Could you check a few things on this model? Use its own coordinates, in mm. Round coordinates to 2 decimals unless told otherwise and drop trailing zeros. Write each loop counter-clockwise with the first axis right and the second up, starting at its lowest first coordinate (ties: lowest second). Pieces come first, ordered by that corner, then holes. Notation, with made-up numbers: (-4, -6.75) -> (39, -6.75) arc R28 ccw to (39, 24.25) -> close; hole circle Ø10 at (-13, -19). An arc over 180 degrees is marked (long way). Return JSON: item names as keys, results as strings.
from build123d import *

# Parameters (mm, degrees)
F0_R     = 1042.9875
F0_R_2   = 6.35
F1_DEPTH = 6.35


with BuildPart() as f1:
    # F0 (on Top) → F1 (new body)
    with BuildSketch(Plane.XY):
        Circle(F0_R)
        with Locations((-534.1764076374, -871.6966720274)):
            Circle(F0_R_2, mode=Mode.SUBTRACT)
        with Locations((-871.6966720274, -534.1764076374)):
            Circle(F0_R_2, mode=Mode.SUBTRACT)
        with Locations((-663.9632122104, -777.4010389312)):
            Circle(F0_R_2, mode=Mode.SUBTRACT)
        with Locations((-777.4010389312, -663.9632122104)):
            Circle(F0_R_2, mode=Mode.SUBTRACT)
        with Locations((-391.2364070784, -944.5282400629)):
            Circle(F0_R_2, mode=Mode.SUBTRACT)
        with Locations((-238.6628677381, -994.1023881186)):
            Circle(F0_R_2, mode=Mode.SUBTRACT)
        with Locations((-80.2126565174, -1019.1984361421)):
            Circle(F0_R_2, mode=Mode.SUBTRACT)
        with Locations((-944.5282400629, -391.2364070784)):
            Circle(F0_R_2, mode=Mode.SUBTRACT)
        with Locations((-994.1023881186, -238.6628677381)):
            Circle(F0_R_2, mode=Mode.SUBTRACT)
        with Locations((-1019.1984361421, -80.2126565174)):
            Circle(F0_R_2, mode=Mode.SUBTRACT)
        with Locations((80.2126565174, -1019.1984361421)):
            Circle(F0_R_2, mode=Mode.SUBTRACT)
        with Locations((238.6628677381, -994.1023881186)):
            Circle(F0_R_2, mode=Mode.SUBTRACT)
        with Locations((391.2364070784, -944.5282400629)):
            Circle(F0_R_2, mode=Mode.SUBTRACT)
        with Locations((534.1764076374, -871.6966720274)):
            Circle(F0_R_2, mode=Mode.SUBTRACT)
        with Locations((663.9632122104, -777.4010389312)):
            Circle(F0_R_2, mode=Mode.SUBTRACT)
        with Locations((777.4010389312, -663.9632122104)):
            Circle(F0_R_2, mode=Mode.SUBTRACT)
        with Locations((871.6966720274, -534.1764076374)):
            Circle(F0_R_2, mode=Mode.SUBTRACT)
        with Locations((944.5282400629, -391.2364070784)):
            Circle(F0_R_2, mode=Mode.SUBTRACT)
        with Locations((994.1023881186, -238.6628677381)):
            Circle(F0_R_2, mode=Mode.SUBTRACT)
        with BuildLine():
            ThreePointArc((1025.5484361421, -80.2126565174), (1018.949136312, -86.5577608975), (1012.8680110729, -79.7144412595))
            ThreePointArc((1012.8680110729, -79.7144412595), (1019.4477359721, -73.8675521372), (1025.5484361421, -80.2126565174))
        make_face(mode=Mode.SUBTRACT)
        with Locations((-1019.1984361421, 80.2126565174)):
            Circle(F0_R_2, mode=Mode.SUBTRACT)
        with Locations((-994.1023881186, 238.6628677381)):
            Circle(F0_R_2, mode=Mode.SUBTRACT)
        with Locations((-944.5282400629, 391.2364070784)):
            Circle(F0_R_2, mode=Mode.SUBTRACT)
        with Locations((-871.6966720274, 534.1764076374)):
            Circle(F0_R_2, mode=Mode.SUBTRACT)
        with Locations((-777.4010389312, 663.9632122104)):
            Circle(F0_R_2, mode=Mode.SUBTRACT)
        with Locations((-663.9632122104, 777.4010389312)):
            Circle(F0_R_2, mode=Mode.SUBTRACT)
        with Locations((-534.1764076374, 871.6966720274)):
            Circle(F0_R_2, mode=Mode.SUBTRACT)
        with Locations((-391.2364070784, 944.5282400629)):
            Circle(F0_R_2, mode=Mode.SUBTRACT)
        with Locations((-238.6628677381, 994.1023881186)):
            Circle(F0_R_2, mode=Mode.SUBTRACT)
        with Locations((-80.2126565174, 1019.1984361421)):
            Circle(F0_R_2, mode=Mode.SUBTRACT)
        with BuildLine():
            ThreePointArc((988.3376139297, 77.7838571352), (990.6294213476, 38.9219359697), (991.39375, 0))
            ThreePointArc((991.39375, 0), (990.6294213476, -38.9219359697), (988.3376139297, -77.7838571352))
            ThreePointArc((988.3376139297, -77.7838571352), (-991.39375, 0), (988.3376139297, 77.7838571352))
        make_face(mode=Mode.SUBTRACT)
        with BuildLine():
            ThreePointArc((1025.5484361421, 80.2126565174), (1019.4477359721, 73.8675521372), (1012.8680110729, 79.7144412595))
            ThreePointArc((1012.8680110729, 79.7144412595), (1018.949136312, 86.5577608975), (1025.5484361421, 80.2126565174))
        make_face(mode=Mode.SUBTRACT)
        with Locations((994.1023881186, 238.6628677381)):
            Circle(F0_R_2, mode=Mode.SUBTRACT)
        with Locations((944.5282400629, 391.2364070784)):
            Circle(F0_R_2, mode=Mode.SUBTRACT)
        with Locations((80.2126565174, 1019.1984361421)):
            Circle(F0_R_2, mode=Mode.SUBTRACT)
        with Locations((238.6628677381, 994.1023881186)):
            Circle(F0_R_2, mode=Mode.SUBTRACT)
        with Locations((391.2364070784, 944.5282400629)):
            Circle(F0_R_2, mode=Mode.SUBTRACT)
        with Locations((777.4010389312, 663.9632122104)):
            Circle(F0_R_2, mode=Mode.SUBTRACT)
        with Locations((663.9632122104, 777.4010389312)):
            Circle(F0_R_2, mode=Mode.SUBTRACT)
        with Locations((871.6966720274, 534.1764076374)):
            Circle(F0_R_2, mode=Mode.SUBTRACT)
        with Locations((534.1764076374, 871.6966720274)):
            Circle(F0_R_2, mode=Mode.SUBTRACT)
    extrude(amount=F1_DEPTH)


solid = f1.part
1) I want a section at C-C, the plane z = 2.5. Count the separate pieces of the cut face and the enclosed holes in it, and give its area (3 significant figures).
Return value:
{"separate pieces": "1", "enclosed holes": "41", "area": "325,000 mm²"}
2) Will these pins go through, and if not, where does the flat tip stop? pin 1 Ø10 at (x, y) = (-80.21, 1019.2) entering from -Z; pin 2 Ø1 at (y, z) = (-499, 4) entering from -X.
Return value:
{"pin 1": "through", "pin 2": "x = -916.14"}
3) I want a section at A-A, the plane y = 0. Please give me the cut outline in (x, z), and give its area (3 significant figures).
Return value:
{"outline": "(-1042.99, 0) -> (-991.39, 0) -> (-991.39, 6.35) -> (-1042.99, 6.35) -> close; (991.39, 0) -> (1042.99, 0) -> (1042.99, 6.35) -> (991.39, 6.35) -> close", "area": "655 mm²"}
4) If I drill on probe 1 along X at (y, z) = (30, 5.75); probe 2 along Y at (x, z) = (78.5, 1.5); probe 3 along X at (y, z) = (-238, 1.5), over which ranges is the centre line in solid material (lowest first)? Write a range as [from, to].
Return value:
{"probe 1": "[-1042.56, -990.94], [990.94, 1042.56]", "probe 2": "[-1040.03, -1025.31], [-1013.08, -988.28], [988.28, 1013.08], [1025.31, 1040.03]", "probe 3": "[-1015.47, -1000.42], [-987.79, -962.4], [962.4, 987.79], [1000.42, 1015.47]"}
5) Thinking about a two-plate mould opening in X: for faces 1 (the face through (-214.91, 967.82, 3.13)), 2 (the face through (922, -381, 0)), 3 (the face through (994.824, 313.285, 3.131)), which applies, pulls with the +X half, pulls with the -X half, needs draft (parallel to the pull), parting line crosses it, or undercut?
Return value:
{"face 1": "undercut", "face 2": "needs draft", "face 3": "parting line crosses it"}
